Autodesk Inventor part; units mm, degrees
ref_plane "YZ Plane" through (0, 0, 0) normal (1, 0, 0) x (0, 1, 0)
ref_plane "XZ Plane" through (0, 0, 0) normal (0, 1, 0) x (-1, 0, 0)
ref_plane "XY Plane" through (0, 0, 0) normal (0, 0, 1) x (1, 0, 0)
sketch "Sketch1" plane through (0, 0, 0) normal (1, 0, 0) x (0, 1, 0)
  line L0 (-40, 84) -> (40, 84)
  line L1 (40, 84) -> (40, -84)
  line L2 (40, -84) -> (-40, -84)
  line L3 (-40, -84) -> (-40, 84)
  line L4 (-40, 84) -> (40, -84) construction
  line L5 (40, 84) -> (-40, -84) construction
  circle A0 centre (5, 0) radius 17.5
  point P0 (0, 0)
  dimension "d0" = 35
  dimension "d5" = 35
  dimension "d6" = 80
  dimension "d7" = 168
  dimension "d8" = 84
extrude "Extrusion1" add sketch "Sketch1" along normal blind 3
sketch "Sketch2" plane through (3, 0, 0) normal (1, 0, 0) x (0, 0, -1)
  circle A0 centre (0, 5) radius 17.5
  circle A1 centre (0, 5) radius 21.5 construction
  line L0 (0, -66.71) -> (0, 54.4228) construction
  line L1 (0, 5) -> (51.042, 5) construction
  point P0 (0, 0)
  point P1 (21.5, 5)
  point P2 (-10.75, 23.6195)
  point P3 (-10.75, -13.6195)
  dimension "d11" = 43
  dimension "d14" = 360
hole "Hole1" at (3, 5, -21.5) at (3, 23.6195, 10.75) at (3, -13.6195, 10.75) direction (-1, 0, 0) diameter 3 depth 10 tip angle 118
sketch "Sketch5" plane through (3, 0, 0) normal (1, 0, 0) x (0, 0, -1)
  circle A0 centre (0, 5) radius 17.5
  circle A1 centre (0, 5) radius 31 construction
  line L0 (-114, -127.2132) -> (84, 27.4814)
  line L1 (84, -40) -> (84, 40)
  line L2 (-84, -40) -> (84, -40)
  line L3 (-112.153, -129.5772) -> (84, 23.6743)
  line L4 (76.1199, 17.5177) -> (74.2729, 19.8817)
  line L5 (64.2997, 8.2828) -> (62.4527, 10.6468)
  line L6 (-84, 40) -> (-84, -40)
  line L7 (-114, -55.0733) -> (-87, -33.9786)
  line L8 (-112.153, -129.5772) -> (-114, -127.2132)
  line L9 (-114, -127.2132) -> (-114, -55.0733)
  line L10 (84, 40) -> (-84, 40)
  line L11 (38.2954, -12.034) -> (36.4484, -9.67)
  line L12 (50.1155, -2.7991) -> (48.2686, -0.4351)
  line L13 (12.291, -32.3509) -> (10.444, -29.9868)
  line L14 (24.1112, -23.116) -> (22.2642, -20.7519)
  line L15 (-84, -33.9786) -> (-87, -33.9786)
  line L16 (-87, -33.9786) -> (-87, 40) construction
  line L17 (-84, 40) -> (-87, 40) construction
  point P0 (0, 0)
  point P1 (11.0887, -29.6815)
  point P2 (12.9357, -32.0456)
  point P3 (2.5006, -40)
  dimension "d24" = 62
  dimension "d25" = 38
  dimension "d27" = 3
  dimension "d28" = 10
  dimension "d33" = 30
  dimension "d37" = 15
  dimension "d40" = 3
  dimension "d43" = 33
  dimension "d54" = 3
  dimension "d56" = 55
extrude "Extrusion2" cut sketch "Sketch5" against normal blind 10 contours L0 L14 L3 L13 | L0 L12 L3 L11 | L0 L4 L3 L5
extrude "Extrusion3" add sketch "Sketch5" against normal up to surface (3 mm away) contours L2 L3 L8 L0 | L0 L9 L7 L15 L6 L2
fillet "Fillet1" radius 10 1 edges at (1.5, -55.0733, 114)
sketch "Sketch8" plane through (3, 0, 0) normal (1, 0, 0) x (0, 0, -1)
  line L0 (84, -25) -> (87, -25)
  line L1 (87, -25) -> (87, -10)
  line L2 (87, -10) -> (84, -10)
  line L3 (84, -10) -> (84, -25)
  line L4 (84, -40) -> (84, 40)
  line L5 (84, -40) -> (84, 40)
  line L6 (84, 0) -> (0, 0) construction
  line L7 (84, 25) -> (87, 25)
  line L8 (87, 25) -> (87, 10)
  line L9 (87, 10) -> (84, 10)
  line L10 (84, 10) -> (84, 25)
  line L11 (84, 40) -> (-84, 40) construction
  line L12 (0, 40) -> (0, 0) construction
  line L13 (-84, -25) -> (-87, -25)
  line L14 (-87, -25) -> (-87, -10)
  line L15 (-87, -10) -> (-84, -10)
  line L16 (-84, -10) -> (-84, -25)
  line L17 (-87, 25) -> (-87, 10)
  line L18 (-87, 10) -> (-84, 10)
  line L19 (-84, 25) -> (-87, 25)
  line L20 (-84, 10) -> (-84, 25)
  line L21 (69, -40) -> (54, -40)
  line L22 (54, -40) -> (54, -43)
  line L23 (54, -43) -> (69, -43)
  line L24 (69, -43) -> (69, -40)
  line L25 (2.5006, -40) -> (84, -40)
  point P0 (-84, 0)
  dimension "d57" = 3
  dimension "d58" = 15
  dimension "d59" = 15
  dimension "d62" = 3
  dimension "d63" = 15
  dimension "d64" = 15
extrude "Extrusion5" add sketch "Sketch8" against normal up to surface (3 mm away)
equation "\"d8\" = 0.5 * d7"
properties part number "Soporte_Rodamientos"
The listing builds one solid part. Answer for the finished solid, in the listing's coordinates (mm). A direction names the side the tool comes from. Coordinates: 2 decimals unless noted, no trailing zeros. Loops run counter-clockwise (first coordinate to the right, second up) from the corner with the lowest first, then second, coordinate; pieces in that order, holes last. Notation, with made-up numbers: (74, 65.5) -> (90, 65.5) arc R26 ccw to (90, 91.5) -> close; hole circle Ø5 at (-36, 7). An arc over 180 degrees is marked (long way). Return JSON: item names as keys, results as strings. Group by question number.
(1) Which of the six approach directions +Z, -Z, +X, -X, +Y, -Y give full straight-line access (tool end or side, diameter ignored) to faces 4 (the flat face through (3, -27, 37)), 5 (the flat face through (1.5, -7.5, -44.1))?
(2) Find the intervals of material crossed by probe 1 along Y at (x, z) = (0.85, 10.75); probe 2 along Y at (x, z) = (2.7, 84.5); probe 3 along Z at (x, y) = (0.7, 29), in increasing order. Write a range as from..to.
(3) A cutting plane is placed at A-A on z = 4. Write down the section's boundary in (x, y).
(4) Given pin 1 Ø1.5 at (x, y) = (2, -41.5) entering from -Z; pin 2 Ø2 at (y, z) = (-7.5, -10.5) entering from +X; pin 3 Ø1.5 at (x, z) = (1.5, -85.5) entering from +Y; pin 4 Ø0.9 at (x, z) = (1.5, -86) entering from -Y, each flat-ended and moving along its own axis, determine where each tip first touches the part or whether it passes through.
(5) A cutting plane is placed at C-C on x = 1.35. Count the separate pieces of the cut face and the enclosed holes in it, and give its area (3 significant figures).
(6) A cutting plane is placed at D-D on z = 54.5. Write down the section's boundary in (x, y).
(7) Determine the mould class of faces 1 (the flat face through (0, -27, 37)), 2 (the flat face through (1.52, 15.2, -68.28)), 3 (the flat face through (1.52, -43.15, 98.74)) for opening direction Y: released by +Y, released by -Y, zero draft, split by the parting line, or undercut.
(8) A cutting plane is placed at B-B on y = -64.5. Write down the section's boundary in (x, z), and give its area (3 significant figures).
The answers:
{
 "1": {"face 4": "+Z, -Z, +X, +Y, -Y", "face 5": "+X, -X"},
 "2": {"probe 1": "y = -50.35..-15.12, -12.12..-8.81, 18.81..22.12, 25.12..40", "probe 2": "y = -107.97..-33.98, -25..-10, 10..25", "probe 3": "z = -84..84"},
 "3": {"outline": "(0, -45.08) -> (3, -45.08) -> (3, -12.04) -> (0, -12.04) -> close; (0, 22.04) -> (3, 22.04) -> (3, 40) -> (0, 40) -> close"},
 "4": {"pin 1": "stops at z = -69", "pin 2": "passes through", "pin 3": "stops at y = 25", "pin 4": "stops at y = -25"},
 "5": {"separate pieces": "1", "enclosed holes": "7", "area": "17,700 mm^2"},
 "6": {"outline": "(0, -84.53) -> (3, -84.53) -> (3, 40) -> (0, 40) -> close"},
 "7": {"face 1": "zero draft", "face 2": "undercut", "face 3": "released by +Y"},
 "8": {"outline": "(0, 28.86) -> (3, 28.86) -> (3, 114) -> (0, 114) -> close", "area": "255 mm^2"}
}
